Read the model definition and answer for the solid it produces. Units are mm, in the model's axes. A direction names the side the tool comes from. Coordinates: 2 decimals unless noted, no trailing zeros. Loops run counter-clockwise (first coordinate to the right, second up) from the corner with the lowest first, then second, coordinate; pieces in that order, holes last. Notation, with made-up numbers: (5, 6) -> (25, 6) arc R14 cw to (25, 24) -> close; hole circle Ø1 at (-35.5, 27.25). An arc over 180 degrees is marked (long way). Answer as a JSON object with one key per item and string values. Group by question number.
1) Flat-ended cylindrical pins translate along their axes: P1, Ø8.5, axis at x = 0, y = -38.1, coming from the -Z side (3 decimals); P2, Ø3, axis at x = -4.5, z = -3, coming from the -Y side; P3, Ø10, axis at x = 0, y = -12.7, coming from the +Z side. Find the tip coordinate at first contact, or state that the pin passes through.
2) Determine the mould class of faces 5 (the face through (-9, 0, 0)), 6 (the face through (0, -25, 9.525)), 7 (the face through (0, -25, 7.938)) for opening direction Z: released by +Z, released by -Z, zero draft, split by the parting line, or undercut.
3) Section B-B, the plane z = 0 is taken. Count the separate pieces of the cut face and the enclosed holes in it, plus the area to 3 significant figures.
4) Section D-D, the plane x = 4.75 is taken. Give the vertices of the cut face in (y, z) (1 decimal), plus the area to 3 significant figures.
5) Which of the six approach directions +Z, -Z, +X, -X, +Y, -Y give full straight-line access (tool end or side, diameter ignored) to faces 1 (the face through (-8.72, -27.762, -1.811)), 2 (the face through (-6.057, -36.193, 8.72)), 3 (the face through (8.72, -19.056, 0.279)), 4 (the face through (0, -25, -7.938))?
6) Consider probe 1 along Y at (x, z) = (0, -8.95) (3 decimals); probe 2 along Y at (x, z) = (0, 8.5); probe 3 along Z at (x, y) = (4, -18) (1 decimal). Determine where each line is inside the solid, lowest interval first. Write a range as [from, to].
from build123d import *

# Parameters (mm, degrees)
F0_W     = 19.05
F0_H     = 19.05
F0_W_2   = 15.875
F0_H_2   = 15.875
F1_DEPTH = 50.8
F3_D     = 5.953125
F3_DEPTH = 6.35
F5_D     = 12.7
F5_DEPTH = 6.35
F7_D     = 12.7
F7_DEPTH = 6.35
F9_D     = 6.35
F9_DEPTH = 6.35


with BuildPart() as f1:
    # F0 (on Front) → F1 (new body)
    with BuildSketch(Plane.XZ):
        Rectangle(F0_W, F0_H)
        Rectangle(F0_W_2, F0_H_2, mode=Mode.SUBTRACT)
    extrude(amount=F1_DEPTH)

    # F3
    with Locations(Plane(origin=(-9.525, 0, 0), x_dir=(0, -1, 0), z_dir=(-1, 0, 0))):
        with Locations((25.4, 0)):
            Hole(F3_D / 2, depth=F3_DEPTH)

    # F5
    with Locations(Plane.YZ.offset(9.525)):
        with Locations((-25.4, 0)):
            Hole(F5_D / 2, depth=F5_DEPTH)

    # F7
    with Locations(Plane.XY.offset(9.525)):
        with Locations((0, -12.7), (0, -38.1)):
            Hole(F7_D / 2, depth=F7_DEPTH)

    # F9
    with Locations(Plane(origin=(0, 0, -9.525), x_dir=(1, 0, 0), z_dir=(0, 0, -1))):
        with Locations((0, 12.7), (0, 38.1)):
            Hole(F9_D / 2, depth=F9_DEPTH)


solid = f1.part
Determined:
{
 "1": {"P1": "z = -9.525", "P2": "through", "P3": "z = -7.94"},
 "2": {"face 5": "zero draft", "face 6": "released by +Z", "face 7": "undercut"},
 "3": {"separate pieces": "4", "enclosed holes": "0", "area": "132 mm²"},
 "4": {"outline": "(-50.8, -9.5) -> (0, -9.5) -> (0, -7.9) -> (-50.8, -7.9) -> close; (-50.8, 7.9) -> (-42.3, 7.9) -> (-42.3, 9.5) -> (-50.8, 9.5) -> close; (-33.9, 7.9) -> (-16.9, 7.9) -> (-16.9, 9.5) -> (-33.9, 9.5) -> close; (-8.5, 7.9) -> (0, 7.9) -> (0, 9.5) -> (-8.5, 9.5) -> close", "area": "135 mm²"},
 "5": {"face 1": "+X, -X", "face 2": "+Z", "face 3": "+X", "face 4": "+Y, -Y"},
 "6": {"probe 1": "[-50.8, -41.275], [-34.925, -15.875], [-9.525, 0]", "probe 2": "[-50.8, -44.45], [-31.75, -19.05], [-6.35, 0]", "probe 3": "[-9.5, -7.9], [7.9, 9.5]"}
}
